Source: CAD feature listing. Evaluate the final solid. Frame: model axes, mm. Face numbers are marked on the shaded views. Round coordinates to 2 decimals unless told otherwise and drop trailing zeros. Loops run counter-clockwise (first coordinate to the right, second up) from the corner with the lowest first, then second, coordinate; pieces in that order, holes last. Notation, with made-up numbers: (-18.75, 71.5) -> (34.25, 71.5) arc R17 ccw to (34.25, 96.5) -> close; hole circle Ø1 at (37, 82). An arc over 180 degrees is marked (long way). Write item = value, one per line.
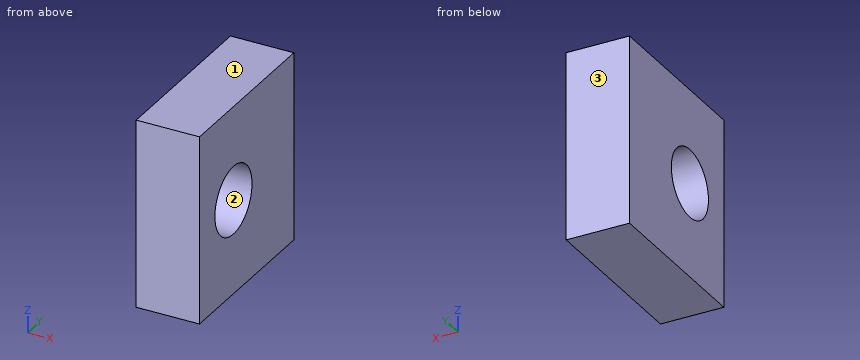
from build123d import *

# Parameters (mm, degrees)
BLOCK_SKETCH_W     = 17.8
BLOCK_SKETCH_H     = 16.4
BLOCK_DEPTH        = 3
TUBE_HOLE_SKETCH_R = 3.225
TUBE_HOLE_DEPTH    = 4


with BuildPart() as part:
    # Block Sketch → Block (new, symmetric)
    with BuildSketch(Plane(origin=(0, 0, 0), x_dir=(0, 0, -1), z_dir=(1, 0, 0))):
        with Locations((0, 90.3)):
            Rectangle(BLOCK_SKETCH_W, BLOCK_SKETCH_H)
    extrude(amount=BLOCK_DEPTH, both=True)

    # Tube Hole Sketch → Tube Hole (cut, symmetric)
    with BuildSketch(Plane(origin=(0, 0, 0), x_dir=(0, 0, -1), z_dir=(1, 0, 0))):
        with Locations(Location((0, 88, 0), (0, 0, 180))):
            Circle(TUBE_HOLE_SKETCH_R)
    extrude(amount=TUBE_HOLE_DEPTH, both=True, mode=Mode.SUBTRACT)


solid = part.part
1. Section query C-C (x = 1.65). Return the cut outline in (y, z) (3 decimals).
Evaluation:
outline = (82.1, -8.9) -> (98.5, -8.9) -> (98.5, 8.9) -> (82.1, 8.9) -> close; hole circle Ø6.45 at (88, 0)
2. Section query A-A (y = 88). Return the cut outline in (x, z) (3 decimals).
Evaluation:
outline = (-3, -8.9) -> (3, -8.9) -> (3, -3.225) -> (-3, -3.225) -> close; (-3, 3.225) -> (3, 3.225) -> (3, 8.9) -> (-3, 8.9) -> close
3. Section query B-B (z = 0). Return the cut outline in (x, y) (3 decimals).
Evaluation:
outline = (-3, 82.1) -> (3, 82.1) -> (3, 84.775) -> (-3, 84.775) -> close; (-3, 91.225) -> (3, 91.225) -> (3, 98.5) -> (-3, 98.5) -> close
4. Mould query, pull axis Z, two halves, no side actions, for the marked faces 1, 2 and 3. Classes: released by +Z, released by -Z, zero draft, split by the parting line, or undercut.
Evaluation:
face_1 = released by +Z
face_2 = undercut
face_3 = zero draft
5. Line query: probe 1 along Y at (x, z) = (-0.75, 0) (3 decimals); probe 2 along Z at (x, y) = (0.55, 88) (3 decimals). Output: solid intervals per line, ascending. Write a range as from..to.
Evaluation:
probe_1 = 82.1..84.775, 91.225..98.5
probe_2 = -8.9..-3.225, 3.225..8.9
